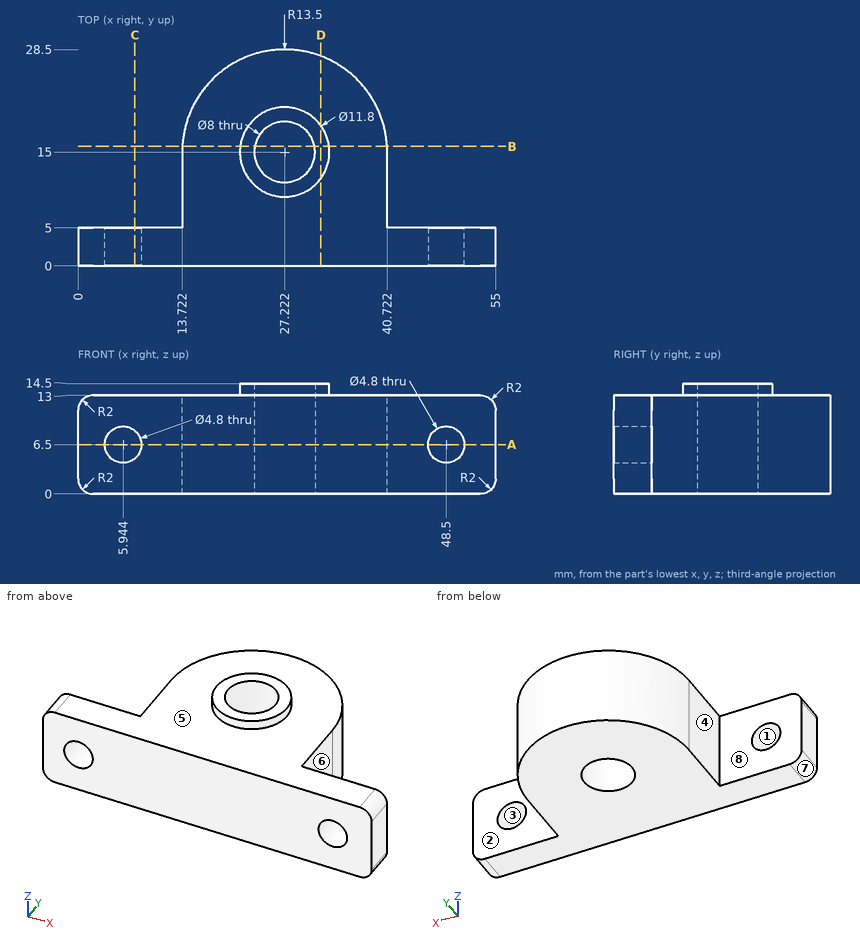
Job drawing, mm, ordinate dimensions from the low corner. One solid piece. A direction names the side the tool comes from. Coordinates: 2 decimals unless noted, no trailing zeros. Order: outer loops, then holes, each group sorted by start corner. A loop starts at its lowest first (then second) coordinate and runs counter-clockwise, first axis right, second up. Notation, with made-up numbers: (79, 81) - (109, 81) arc R12 cw to (109, 98) - close; hole circle Ø4 at (-32, -39.75). An arc over 180 degrees is marked (long way). Return JSON: item names as keys, results as strings. Group by question number.
1) Saw through at A-A, the plane z = 6.5. Write the cut outline in (x, y) (1 decimal), plus the area to 3 significant figures.
2) Flat gauge pins, fed straight in: P1, Ø8, axis at y = 9.5, z = 9, coming from the -X side; P2, Ø1, axis at y = 23, z = 5, coming from the +X side; P3, Ø5.5, axis at x = 48.5, z = 6.5, coming from the -Y side; P4, Ø1, axis at x = 34.5, y = 4, coming from the +Z side. Where does each tip first touch, or does it go through?
3) Mould opens along X. For the marked faces 1, 2, 3 and 4 say: released by +X, released by -X, zero draft, split by the parting line, or undercut.
4) Saw through at B-B, the plane y = 15.75. Write the cut outline in (x, z) (1 decimal), plus the area to 3 significant figures.
5) Tool access for the marked faces 5, 6, 7 and 8: list every direction of +Z, -Z, +X, -X, +Y, -Y with a clear straight run to the whole face (end or side of a thin tool).
6) Saw through at C-C, the plane x = 7.5. Write the cut outline in (y, z).
7) Saw through at D-D, the plane x = 32. Write the cut outline in (y, z).
8) Probe line 1 (X direction, y = 15, z = 5.5); line 2 (X direction, y = 2, z = 7); line 3 (Y direction, x = 50.5, z = 2). List the from-to ranges inside material, lowest first. Write a range as from..to.
Values found:
{
 "1": {"outline": "(0, 0) - (3.5, 0) - (3.5, 5) - (0, 5) - close; (8.3, 0) - (46.1, 0) - (46.1, 5) - (40.7, 5) - (40.7, 15) arc R13.5 ccw to (13.7, 15) - (13.7, 5) - (8.3, 5) - close; (50.9, 0) - (55, 0) - (55, 5) - (50.9, 5) - close; hole circle Ø8 at (27.2, 15)", "area": "733 mm²"},
 "2": {"P1": "stops at x = 13.72", "P2": "stops at x = 38.45", "P3": "stops at y = 0", "P4": "stops at z = 13"},
 "3": {"face 1": "undercut", "face 2": "zero draft", "face 3": "undercut", "face 4": "released by -X"},
 "4": {"outline": "(13.7, 0) - (23.3, 0) - (23.3, 14.5) - (21.4, 14.5) - (21.4, 13) - (13.7, 13) - close; (31.2, 0) - (40.7, 0) - (40.7, 13) - (33.1, 13) - (33.1, 14.5) - (31.2, 14.5) - close", "area": "254 mm²"},
 "5": {"face 5": "+Z", "face 6": "+Z, -Z, +X, +Y", "face 7": "-Z, -X, +Y, -Y", "face 8": "+Z, -Z, -X, +Y"},
 "6": {"outline": "(0, 0) - (5, 0) - (5, 4.67) - (0, 4.67) - close; (0, 8.33) - (5, 8.33) - (5, 13) - (0, 13) - close"},
 "7": {"outline": "(0, 0) - (27.63, 0) - (27.63, 13) - (18.46, 13) - (18.46, 14.5) - (11.54, 14.5) - (11.54, 13) - (0, 13) - close"},
 "8": {"line 1": "x = 13.72..23.22, 31.22..40.72", "line 2": "x = 0..3.6, 8.29..46.15, 50.85..55", "line 3": "y = 0..5"}
}
